Drawing for the job (mm, zero at the part's lowest x, y, z). A direction names the side the tool comes from. Round coordinates to 2 decimals unless told otherwise and drop trailing zeros. Order: outer loops, then holes, each group sorted by start corner. A loop starts at its lowest first (then second) coordinate and runs counter-clockwise, first axis right, second up. Notation, with made-up numbers: (21.25, 84.25) - (46.25, 84.25) arc R18 ccw to (46.25, 100.25) - close; hole circle Ø2 at (34, 38.25). An arc over 180 degrees is marked (long way). Answer as a JSON object with one key per item and string values.
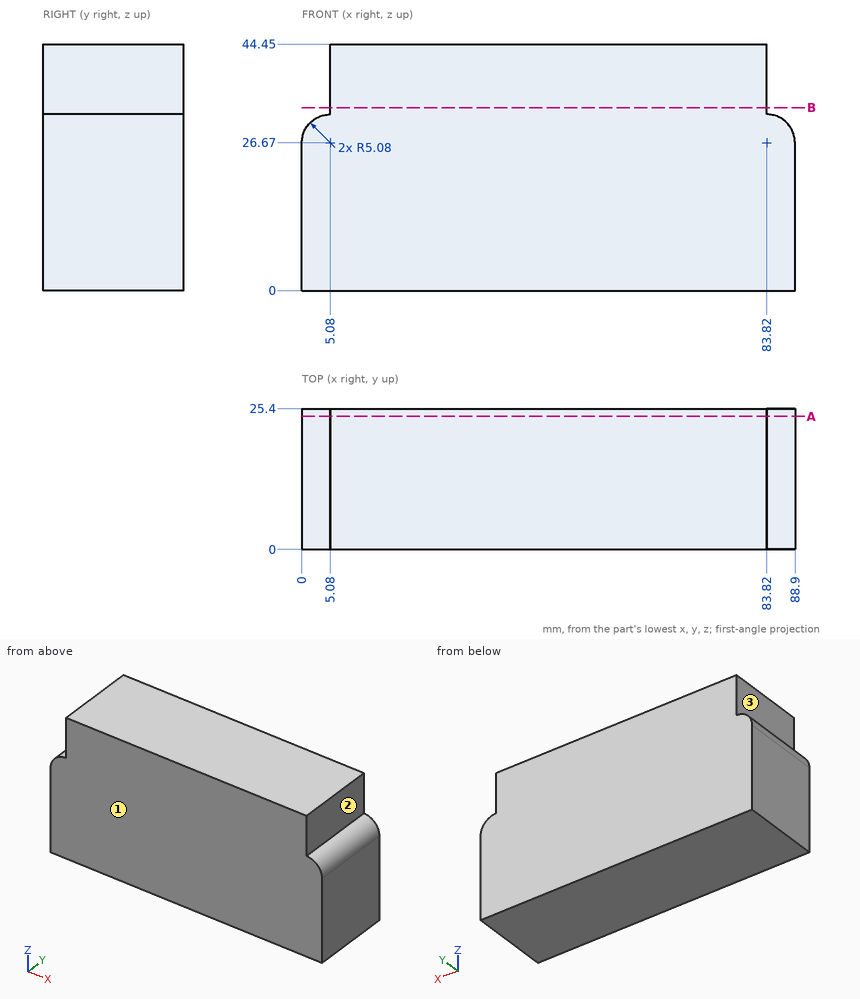
Item 1: Drop flat-ended pins along their axis: P1, Ø14, axis at y = 17, z = 37, coming from the +X side; P2, Ø10, axis at y = 12, z = 36, coming from the -X side; P3, Ø8, axis at y = 15.5, z = 35, coming from the +X side. Give the stop position or say it passes through.
Taken from the geometry:
{"P1": "x = 87.66", "P2": "x = 2.42", "P3": "x = 86.48"}
Item 2: Probe L1, parallel to X at y = 17.25, z = 35; L2, parallel to Z at x = 84, y = 22; L3, parallel to X at y = 7, z = 31. List the from-to ranges inside material, lowest first. Write a range as from..to.
Taken from the geometry:
{"L1": "5.08..83.82", "L2": "0..31.75", "L3": "2.42..86.48"}
Item 3: Cut at A-A (y = 24). Write the cut outline in (x, z), plus the area to 3 significant figures.
Taken from the geometry:
{"outline": "(0, 0) - (88.9, 0) - (88.9, 26.67) arc R5.08 ccw to (83.82, 31.75) - (83.82, 44.45) - (5.08, 44.45) - (5.08, 31.75) arc R5.08 ccw to (0, 26.67) - close", "area": "3,810 mm2"}
Item 4: Tool access for the marked faces 1, 2 and 3: list every direction of +Z, -Z, +X, -X, +Y, -Y with a clear straight run to the whole face (end or side of a thin tool).
Taken from the geometry:
{"face 1": "+Z, -Z, +X, -X, -Y", "face 2": "+Z, +X, +Y, -Y", "face 3": "+Z, -X, +Y, -Y"}
Item 5: Cut at B-B (z = 33). Write the cut outline in (x, y).
Taken from the geometry:
{"outline": "(5.08, 0) - (83.82, 0) - (83.82, 25.4) - (5.08, 25.4) - close"}
